```python
from build123d import *

# Parameters (mm, degrees)
F2_R     = 1.5533685179
F3_DEPTH = 50.8


# Not quite as in the source:
# - a fillet or chamfer that OpenCascade refuses, or shapes differently, is made with other operations: its cross-section is extruded or revolved along the edge and cut away or added


with BuildPart() as f1:
    # F0 (on Top) → F1 (revolve)
    with BuildSketch(Plane.XY):
        Polygon((25.7452992698, 34.3298881523), (0, 0), (0, -48.7618558109), (4.5166942291, -48.7618558109), (4.5166942291, 0), (29.4045954943, 31.4324982464), align=None)
    revolve(axis=Axis((0, -24.3809279054, 0), (0, -1, 0)))

    # F2 (on face) → F3 (cut)
    with BuildSketch(Plane.XZ.offset(48.7618558109)):
        Circle(F2_R)
    extrude(amount=-F3_DEPTH, mode=Mode.SUBTRACT)

    # F4: fillet of radius 5.08 on 1 edges, made by hand

    # F4_s1 → F4_t2 (revolve, cut)
    with BuildSketch(Plane.XY):
        with BuildLine():
            ThreePointArc((25.7452992698, 34.3298881523), (27.3445295723, 30.9972333724), (26.261540234, 27.4629357709))
            Line((26.261540234, 27.4629357709), (26.3411945536, 27.3998663697))
            Line((26.3411945536, 27.3998663697), (29.4842498139, 31.3694288452))
            Line((29.4842498139, 31.3694288452), (29.4676648955, 31.5121525661))
            ThreePointArc((29.4676648955, 31.5121525661), (27.6380167832, 32.960847519), (25.8146287701, 34.4041577987))
            Line((25.8146287701, 34.4041577987), (25.7452992698, 34.3298881523))
        make_face()
    revolve(axis=Axis((0, 31.4324982464, 0), (0, -1, 0)), mode=Mode.SUBTRACT)


solid = f1.part
```
Model file for the job. Use its own axes, mm. Give positions to 0.01 mm unless a question says otherwise; leave off trailing zeros. Order: outer loops, then holes, each group sorted by start corner. A loop starts at its lowest first (then second) coordinate and runs counter-clockwise, first axis right, second up.
1) Mould opens along X. For faces 1 (the flat face through (0, -48.762, -2)), 2 (the cylindrical face through (-1.23, -23.72, -0.95)), 3 (the conical face through (4.94, 7.82, -9.5)), 4 (the conical face through (3.73, 10.78, -7.17)) say: +X half, -X half, draft (parallel to the pull), parting line (faces both ways), or undercut.
2) Saw through at D-D, the plane y = 5.5. Write the cut outline in (x, z).
3) Pin check, flat tips, straight feed: pin 1 (8 mm diameter, centred on x = 0, y = -10, fed in from +Z); pin 2 (2 mm diameter, centred on x = -3.5, y = 24, fed in from -Z); pin 3 (10 mm diameter, centred on y = 16.5, z = -21.5, fed in from -X); pin 4 (8 mm diameter, centred on y = 7.5, z = -16, fed in from +X). Stop position of each tip, or through.
4) Saw through at C-C, the plane y = -32.5. Write the cut outline in (x, z), then the cut area to 3 significant figures.
5) Wall check: probe 1 along Z at (x, y) = (0, -35); probe 2 along Z at (x, y) = (9, 19); probe 3 along X at (y, z) = (14.5, -7). Give the ranges that are in metal, low to high.
Computed:
1. face 1: draft
1. face 2: undercut
1. face 3: parting line
1. face 4: undercut
2. outline: circle Ø17.74 at (0, 0); hole circle Ø8.25 at (0, 0)
3. pin 1: stops at z = 4.52
3. pin 2: stops at z = -24.07
3. pin 3: stops at x = -9.64
3. pin 4: passes through
4. outline: circle Ø9.03 at (0, 0); hole circle Ø3.11 at (0, 0)
4. area: 56.5 mm2
5. probe 1: z = -4.52 to -1.55, 1.55 to 4.52
5. probe 2: z = -17.37 to -11.05, 11.05 to 17.37
5. probe 3: x = -14.38 to -8.32, 8.32 to 14.38
